The listing builds one solid part. Answer for the finished solid, in the listing's coordinates (mm). Face numbers are marked on the shaded views. Coordinates: 2 decimals unless noted, no trailing zeros. Loops run counter-clockwise (first coordinate to the right, second up) from the corner with the lowest first, then second, coordinate; pieces in that order, holes last. Notation, with made-up numbers: M -1,5 L 58,5 A7 cw 58,16 Z; hole C 69,-39.5 d2. An arc over 180 degrees is marked long. Answer as a JSON object with one key per item and string values. Group by question number.
1. A cutting plane is placed at C-C on x = -3.25. Give the vertices of the cut face in (y, z) (3 decimals).
2. Determine the mould class of the marked faces 1 and 2 for opening direction Z: released by +Z, released by -Z, zero draft, split by the parting line, or undercut.
3. A cutting plane is placed at D-D on y = 2.9. Give the vertices of the cut face in (x, z).
4. A cutting plane is placed at A-A on z = 11.5. Give the vertices of the cut face in (x, y) (3 decimals), and give its area (3 significant figures).
5. Given pin 1 (0.8 mm diameter, centred on x = -15.5, y = 2, fed in from -Z); pin 2 (3 mm diameter, centred on y = 2.54, z = -2.54, fed in from +X); pin 3 (3 mm diameter, centred on x = -24.36, z = 3.13, fed in from +Y), each flat-ended and moving along its own axis, determine where each tip first touches the part or whether it passes through.
6. Straight lines are drawn through the part: L1, parallel to X at y = 0.4, z = 14 (3 decimals); L2, parallel to Z at x = -16.25, y = 1.2 (3 decimals); L3, parallel to X at y = 2.3, z = -0.5. For each, find the intervals that lie inside material, in ascending order.
7. A cutting plane is placed at B-B on x = -15.25. Give the vertices of the cut face in (y, z) (3 decimals), and give its area (3 significant figures).
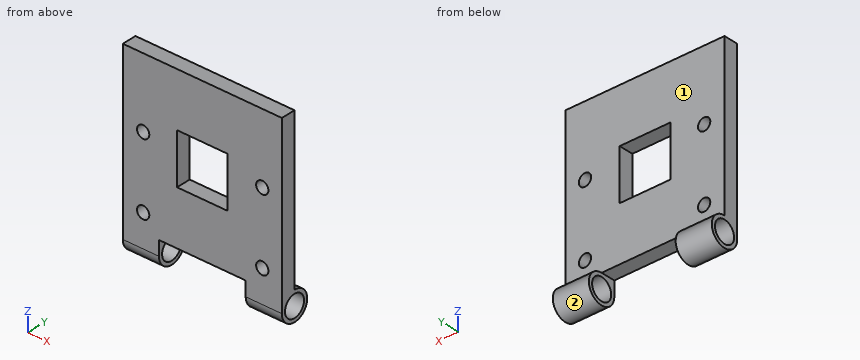
Autodesk Inventor part; units mm, degrees
ref_plane "Work Plane1" through (-6.35, 0, 0) normal (0, 0, -1) x (-1, 0, 0)
ref_plane "YZ Plane" through (0, 0, 0) normal (1, 0, 0) x (0, 1, 0)
ref_plane "XZ Plane" through (0, 0, 0) normal (0, 1, 0) x (-1, 0, 0)
sketch "Sketch1" plane through (0, 0, 0) normal (0, 1, 0) x (-1, 0, 0)
  line L0 (0, 0) -> (27.94, 0)
  line L1 (27.94, 0) -> (27.94, 27.94)
  line L2 (27.94, 27.94) -> (0, 27.94)
  line L3 (0, 27.94) -> (0, 0)
  line L4 (18.415, 18.415) -> (9.525, 18.415)
  line L5 (9.525, 18.415) -> (9.525, 9.525)
  line L6 (9.525, 9.525) -> (18.415, 9.525)
  line L7 (18.415, 9.525) -> (18.415, 18.415)
  line L8 (27.94, 0) -> (18.415, 9.525)
  line L9 (9.525, 18.415) -> (0, 27.94)
  line L10 (27.94, 27.94) -> (18.415, 18.415)
  line L11 (9.525, 9.525) -> (0, 0)
  dimension "d0" = 27.94
  dimension "d1" = 8.89
extrude "Extrusion1" add sketch "Sketch1" along normal blind 2.54 contours L11 L6 L8 L0 | L3 L9 L5 L11 | L8 L7 L10 L1 | L2 L10 L4 L9
sketch "Sketch2" plane through (0, 0, 27.94) normal (1, 0, 0) x (0, 0, -1)
  circle A0 centre (30.48, 2.54) radius 2.54
  line L0 (27.94, 0) -> (30.48, 0)
  line L1 (27.94, 2.5262) -> (27.94, 0)
  circle A1 centre (30.48, 2.54) radius 1.905
  line L2 (0, 0) -> (27.94, 0)
  line L3 (27.94, 0) -> (27.94, 2.54)
  line L4 (27.94, 2.54) -> (27.94, 0)
  line L5 (27.94, 0) -> (30.48, 0)
  line L6 (27.94, 2.54) -> (28.575, 2.54)
  line L7 (28.575, 2.54) -> (28.575, 0)
  line L8 (28.575, 0) -> (27.94, 0)
  line L9 (27.94, 0) -> (27.94, 2.54)
  line L10 (30.48, 0.635) -> (27.94, 0.635)
  line L11 (27.94, 0.635) -> (27.94, 0)
  line L12 (27.94, 0) -> (30.48, 0)
  line L13 (30.48, 0) -> (30.48, 0.635)
  line L14 (28.9005, 1.0162) -> (28.3369, 1.0162)
  line L15 (28.3369, 1.0162) -> (28.3369, 0.4026)
  line L16 (28.3369, 0.4026) -> (28.9005, 0.4026)
  line L17 (28.9005, 0.4026) -> (28.9005, 1.0162)
  dimension "d4" = 5.08
  dimension "d5" = 3.81
sketch "Sketch3" plane through (-27.94, 0, 0) normal (-1, 0, 0) x (0, 0, 1)
  circle A0 centre (-2.54, 2.54) radius 1.905
  circle A1 centre (-2.54, 2.54) radius 2.54
  line L0 (-0.3403, 2.54) -> (-0.3403, 0)
  line L1 (0, 2.54) -> (0, 0)
  line L2 (-0.3403, 0) -> (0, 0)
  line L3 (0, 0) -> (0, 2.54)
  line L4 (0, 2.54) -> (-0.3403, 2.54)
  line L5 (0, 0) -> (-5.4168, 0)
  line L6 (0, 0) -> (0, 2.54)
  line L7 (0, 2.0092) -> (-0.6973, 2.0092)
  line L8 (-0.6973, 2.0092) -> (-0.6973, 0)
  line L9 (-0.6973, 0) -> (0, 0)
  line L10 (0, 0) -> (0, 2.0092)
  line L11 (-2.54, 0.635) -> (0, 0.635)
  line L12 (0, 0.635) -> (0, 0)
  line L13 (0, 0) -> (-2.54, 0)
  line L14 (-2.54, 0) -> (-2.54, 0.635)
  line L15 (-1.27, 1.1201) -> (0, 1.1201)
  line L16 (0, 1.1201) -> (0, 0)
  line L17 (0, 0) -> (-1.27, 0)
  line L18 (-1.27, 0) -> (-1.27, 1.1201)
  point P0 (0, 1.27)
  dimension "d10" = 5.08
  dimension "d11" = 3.81
ref_plane "Work Plane1" through (-6.35, 0, 0) normal (0, 0, -1) x (-1, 0, 0)
sketch "Sketch5" plane through (0, 0, 0) normal (0, -1, 0) x (1, 0, 0)
  circle A0 centre (-24.3621, 3.1287) radius 1.0795
  circle A1 centre (-24.3621, 3.1287) radius 1.0795
  circle A2 centre (-3.4325, 3.1287) radius 1.0795
  circle A3 centre (-3.4325, 15.6763) radius 1.0795
  circle A4 centre (-24.3621, 15.6763) radius 1.0795
  circle A5 centre (-3.4325, 15.6763) radius 1.0795
  circle A6 centre (-3.4325, 3.1287) radius 1.0795
  circle A7 centre (-24.3621, 3.1287) radius 1.0795
  circle A8 centre (-24.3621, 15.6763) radius 1.0795
  point P0 (0, 0)
extrude "Extrusion5" cut sketch "Sketch5" against normal blind 6.0325
extrude "Extrusion6" add sketch "Sketch2" against normal blind 6.35 contours A0 L13 A1 L6 | L6 L7 L14 A0 | L0 L7 L16 L17 A0 | A0 L17 L10 L13 | A0 L14 L15 L10 L1 | A1 L10 L17 L14 L7 | L17 L16 L7 L10 A0 | A0 L10 L17 | L0 L1 L10 L15 L16 L7 | L14 L7 A0 | A0 L7 L10 L15 L14 | L14 L17 L10 A0 L7 | L10 L7 A0 | L16 L15 L10 L7
extrude "Extrusion7" add sketch "Sketch3" against normal blind 6.35 contours A0 L14 A1 L4 L0 L7 L8 L15 | A0 L18 L11 | L11 L18 A1 L14 | L15 L8 A1 L11 L18 | L11 A1 L18 | A1 L18 L5 | L15 A1 L8 | L8 L7 L0 A1 L15 | L11 L8 L5 L18 A1 | A1 L8 L11 | A1 L7 L0 L4 | A1 L15 L0 L11 L8 | A1 L0 L15 | L11 L0 L5 L8 | L7 L1 L15 L0 A1 | A1 L0 L7 | L15 L1 L11 L0 | L11 L1 L2 L0
properties part number "Top of the cam case (real version)"
From the geometry:
{
 "1": {"outline": "M 0,-2.54 A2.54 ccw long 2.54,0 L 2.54,2.065 L 0,2.065 Z; M 0,4.193 L 2.54,4.193 L 2.54,14.612 L 0,14.612 Z; M 0,16.74 L 2.54,16.74 L 2.54,27.94 L 0,27.94 Z; hole C 2.54,-2.54 d3.81"},
 "2": {"face 1": "zero draft", "face 2": "split by the parting line"},
 "3": {"outline": "M -27.94,-5.05 L -21.59,-5.05 L -21.59,-4.41 L -27.94,-4.41 Z; M -27.94,-0.67 L -21.59,-0.67 L -21.59,-0.03 L -27.94,-0.03 Z; M -6.35,-5.05 L 0,-5.05 L 0,-4.41 L -6.35,-4.41 Z; M -6.35,-0.67 L 0,-0.67 L 0,-0.03 L -6.35,-0.03 Z"},
 "4": {"outline": "M -27.94,0 L -18.415,0 L -18.415,2.54 L -27.94,2.54 Z; M -9.525,0 L 0,0 L 0,2.54 L -9.525,2.54 Z", "area": "48.4 mm²"},
 "5": {"pin 1": "stops at z = 0", "pin 2": "passes through", "pin 3": "stops at y = 2.54"},
 "6": {"L1": "x = -27.94 to -18.415, -9.525 to 0", "L2": "z = 0 to 9.525, 18.415 to 27.94", "L3": "x = -27.94 to -21.59, -6.35 to 0"},
 "7": {"outline": "M 0,0 L 2.54,0 L 2.54,9.525 L 0,9.525 Z; M 0,18.415 L 2.54,18.415 L 2.54,27.94 L 0,27.94 Z", "area": "48.4 mm²"}
}
